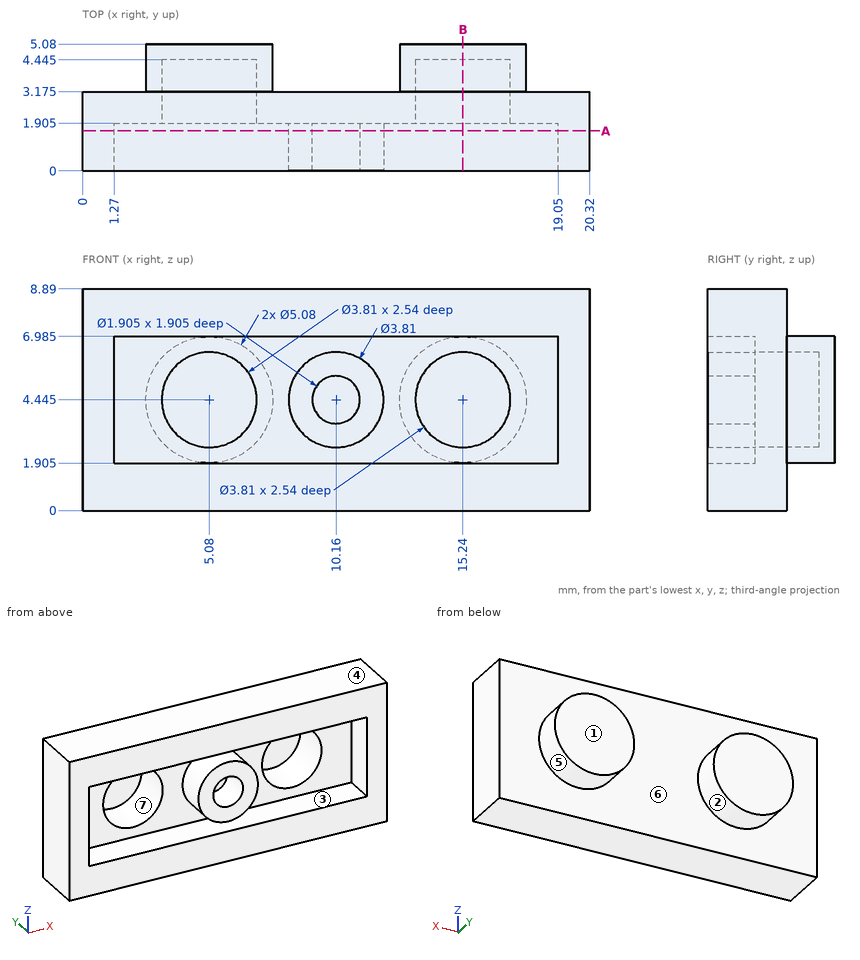
Verification items for this drawing (mm, ordinates from the low corner). A direction names the side the tool comes from. Coordinates: 2 decimals unless noted, no trailing zeros. Order: outer loops, then holes, each group sorted by start corner. A loop starts at its lowest first (then second) coordinate and runs counter-clockwise, first axis right, second up. Notation, with made-up numbers: M 56,11.25 L 105,11.25 A15 ccw 105,16.25 Z; hole C -16.5,87 d9. An arc over 180 degrees is marked long. One line per item, written item: value. Start each with the question number.
Item 1: Mould release check, pull along Z, two halves, no side actions. Record for the marked faces 4, 5, 6 and 7: pulls with the +Z half, pulls with the -Z half, needs draft (parallel to the pull), parting line crosses it, or undercut.
Item 2: Access from +Z, -Z, +X, -X, +Y, -Y to the whole of each face (thin tool, end or side, straight path). Record for the marked faces 1, 2 and 3.
Item 3: Sectioned sample at A-A on y = 1.6. Give the number of separate pieces and of enclosed holes in the cut face, then the cut area to 3 significant figures.
Item 4: Thickness scan on probe 1 along Z at (x, y) = (13, 0.85) (3 decimals); probe 2 along Z at (x, y) = (15.24, 3.5) (3 decimals); probe 3 along X at (y, z) = (0.65, 4.25) (3 decimals). Record the ranges inside material, lowest first.
Item 5: Sectioned sample at B-B on x = 15.24. Record the cut outline in (y, z) (3 decimals).
Item 6: Depth check by flat-ended pin: P1, Ø1.9, axis at x = 14.5, z = 4, coming from the -Y side (3 decimals); P2, Ø2.5, axis at x = 11.5, z = 3, coming from the +Y side (3 decimals); P3, Ø4.5, axis at x = 15.24, z = 4.445, coming from the -Y side (3 decimals). Enter the tip coordinate at first touch or a pass-through.
Calculated:
1. face 4: pulls with the +Z half
1. face 5: parting line crosses it
1. face 6: needs draft
1. face 7: undercut
2. face 1: +Z, -Z, +X, -X, +Y
2. face 2: +Y
2. face 3: -Y
3. separate pieces: 2
3. enclosed holes: 2
3. area: 98.9 mm^2
4. probe 1: 0 to 1.905, 6.985 to 8.89
4. probe 2: 1.905 to 2.54, 6.35 to 6.985
4. probe 3: 0 to 1.27, 8.265 to 9.228, 11.092 to 12.055, 19.05 to 20.32
5. outline: M 0,0 L 3.175,0 L 3.175,1.905 L 5.08,1.905 L 5.08,6.985 L 3.175,6.985 L 3.175,8.89 L 0,8.89 L 0,6.985 L 1.905,6.985 L 1.905,6.35 L 4.445,6.35 L 4.445,2.54 L 1.905,2.54 L 1.905,1.905 L 0,1.905 Z
6. P1: y = 4.445
6. P2: y = 3.175
6. P3: y = 1.905
